Geometry: final body of the model. Coordinates: model frame, mm. Face numbers are marked on the shaded views. A direction names the side the tool comes from. Give positions to 0.01 mm unless a question says otherwise; leave off trailing zeros. Order: outer loops, then holes, each group sorted by start corner. A loop starts at its lowest first (then second) coordinate and runs counter-clockwise, first axis right, second up. Notation, with made-up numbers: (53.5, -0.5) -> (80.5, -0.5) arc R11 cw to (80.5, 3.5) -> close; hole circle Ø6 at (42.5, -27.75). An arc over 180 degrees is marked (long way). Answer in a Markdown table with one row per item. Add a question column.
Q1. Set-up query: the marked faces 1, 2, 3, 4 and 5. Return all of +Z, -Z, +X, -X, +Y, -Y with unobstructed straight access to the full face (end or side cutting, diameter ignored); none if empty.
Q2. Cut plane A-A on y = 0. Return the cut outline in (x, z).
Q3. Contact query for flat-ended pins moving along their axis: P1, Ø0.8, axis at x = 12, z = 0.5, coming from the -Y side (3 decimals); P2, Ø5, axis at x = -6, y = -8.5, coming from the +Z side; P3, Ø5, axis at x = -21.92, y = 0, coming from the +Z side; P4, Ø8, axis at x = -9, y = 2.5, coming from the -Z side. Output: stop coordinate, or through.
Q4. Cut plane B-B on x = 0. Return the cut outline in (y, z).
Q5. Cut plane C-C on y = 11. Return the cut outline in (x, z) (3 decimals).
Q6. Line query: line 1 along Y through (x, z) = (0, 0.65); line 2 along X through (y, z) = (14, 0.8) (3 decimals); line 3 along Z through (x, y) = (-16, 3). Output: solid intervals per line, ascending. Write a range as from..to.
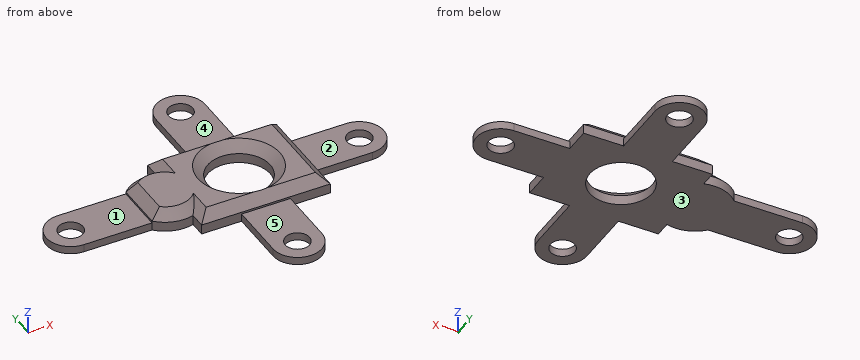
from build123d import *

# Parameters (mm, degrees)
F0_R         = 4.064
F1_DEPTH     = 2.54
F0_R_2       = 1.5875
F2_DEPTH     = 1.016
F3_T1_DEPTH  = 23.2960747894
F3_T3_DEPTH  = 19.6130747894
F3_T5_DEPTH  = 12.8820747894
F3_T10_DEPTH = 8.6144406225
F3_S11_R     = 4.6355
F3_T12_DEPTH = 6
F3_T16_ANGLE = 143.4241535748
F3_T21_ANGLE = 143.4241535748
F3_T26_DEPTH = 8.6144406225
F3_S27_R     = 4.6355
F3_T28_DEPTH = 6
F3_T35_ANGLE = 143.4241535748
F3_T39_DEPTH = 8.6144406225
F3_S40_R     = 4.6355
F3_T41_DEPTH = 6
F3_T47_DEPTH = 8.6144406225
F3_S48_R     = 4.6355
F3_T49_DEPTH = 6
F3_T52_ANGLE = 143.4241535748


# Not quite as in the source:
# - a fillet or chamfer that OpenCascade refuses, or shapes differently, is made with other operations: its cross-section is extruded or revolved along the edge and cut away or added
# - a feature names something its author has since deleted; it is built from what else it names


with BuildPart() as f1:
    # F0 (on Top) → F1 (new body)
    with BuildSketch(Plane.XY):
        Polygon((-8.382, 6.5405), (-8.382, 4.4581341669), (-8.382, -4.4581341669), (-8.382, -6.5405), (-3.175, -6.5405), (3.175, -6.5405), (8.382, -6.5405), (8.382, -3.175), (8.382, 3.175), (8.382, 6.5405), (3.175, 6.5405), (-3.175, 6.5405), align=None)
        Circle(F0_R, mode=Mode.SUBTRACT)
        with BuildLine():
            Line((-8.382, -4.4581341669), (-8.382, 4.4581341669))
            ThreePointArc((-8.382, 4.4581341669), (-10.8856754478, 4.4683224077), (-13.0294598813, 3.175))
            Line((-13.0294598813, 3.175), (-13.0294598813, -3.175))
            ThreePointArc((-13.0294598813, -3.175), (-10.8856754478, -4.4683224077), (-8.382, -4.4581341669))
        make_face()
    extrude(amount=F1_DEPTH)

    # F0 (on Top) → F2 (join)
    with BuildSketch(Plane.XY):
        with BuildLine():
            Line((-13.0294598813, -3.175), (-13.0294598813, 3.175))
            Line((-13.0294598813, 3.175), (-21.9194598813, 3.175))
            ThreePointArc((-21.9194598813, 3.175), (-25.0944598813, 0), (-21.9194598813, -3.175))
            Line((-21.9194598813, -3.175), (-13.0294598813, -3.175))
        make_face()
        with Locations((-21.9194598813, 0)):
            Circle(F0_R_2, mode=Mode.SUBTRACT)
        with BuildLine():
            Line((3.175, -6.5405), (-3.175, -6.5405))
            Line((-3.175, -6.5405), (-3.175, -14.1605))
            ThreePointArc((-3.175, -14.1605), (0, -17.3355), (3.175, -14.1605))
            Line((3.175, -14.1605), (3.175, -6.5405))
        make_face()
        with Locations((0, -14.1605)):
            Circle(F0_R_2, mode=Mode.SUBTRACT)
        with BuildLine():
            Line((-3.175, 14.1605), (-3.175, 6.5405))
            Line((-3.175, 6.5405), (3.175, 6.5405))
            Line((3.175, 6.5405), (3.175, 14.1605))
            ThreePointArc((3.175, 14.1605), (0, 17.3355), (-3.175, 14.1605))
        make_face()
        with Locations((0, 14.1605)):
            Circle(F0_R_2, mode=Mode.SUBTRACT)
        with BuildLine():
            Line((15.6725401187, 3.175), (8.382, 3.175))
            Line((8.382, 3.175), (8.382, -3.175))
            Line((8.382, -3.175), (15.6725401187, -3.175))
            ThreePointArc((15.6725401187, -3.175), (18.8475401187, 0), (15.6725401187, 3.175))
        make_face()
        with Locations((15.6725401187, 0)):
            Circle(F0_R_2, mode=Mode.SUBTRACT)
    extrude(amount=F2_DEPTH)

    # F3: chamfer of 1.27 on 9 edges, made by hand

    # F3_s2 → F3_t1 (cut)
    with BuildSketch(Plane.YZ.offset(-11.6480373947)):
        Polygon((-5.2705, 2.54), (-6.5405, 1.27), (-6.5405, 2.54), align=None)
        Polygon((6.5405, 1.27), (5.2705, 2.54), (6.5405, 2.54), align=None)
    extrude(amount=F3_T1_DEPTH, mode=Mode.SUBTRACT)

    # F3_s4 → F3_t3 (cut)
    with BuildSketch(Plane.XZ.offset(-9.8065373947)):
        Polygon((7.112, 2.54), (8.382, 1.27), (8.382, 2.54), align=None)
    extrude(amount=F3_T3_DEPTH, mode=Mode.SUBTRACT)

    # F3_s6 → F3_t5 (cut)
    with BuildSketch(Plane.XZ.offset(-6.4410373947)):
        Polygon((-11.7594598813, 2.54), (-13.0294598813, 1.27), (-13.0294598813, 2.54), align=None)
    extrude(amount=F3_T5_DEPTH, mode=Mode.SUBTRACT)


with BuildPart() as f3_tool8:
    # F3_s9 → F3_t10 (new body)
    with BuildSketch(Plane.XZ.offset(1.1920967722)):
        Polygon((-7.112, 2.54), (-8.382, 1.27), (-8.382, 2.54), align=None)
    extrude(amount=F3_T10_DEPTH)

    # F3_s11 → F3_t12 (cut, symmetric)
    with BuildSketch(Plane.XY.offset(1.9)):
        with Locations((-9.652, 0)):
            Circle(F3_S11_R)
    extrude(amount=F3_T12_DEPTH, both=True, mode=Mode.SUBTRACT)


with BuildPart() as f1_1:
    add(f1.part)

    # F3_t7: cut F3_tool8
    add(f3_tool8.part, mode=Mode.SUBTRACT)


with BuildPart() as f3_tool14:
    # F3_s15 → F3_t16 (revolve)
    with BuildSketch(Plane(origin=(-0.0239192805, 0.47989245, 0), x_dir=(0, 0, 1), z_dir=(-0.0497812044, 0.9987601472, 0))):
        Polygon((2.54, -13.005532941), (1.27, -14.275532941), (2.54, -14.275532941), align=None)
    revolve(axis=Axis((-9.652, 0, 2.54), (0, 0, 1)), revolution_arc=F3_T16_ANGLE)

    split(bisect_by=Plane.YZ.offset(-8.382), keep=Keep.BOTTOM)


with BuildPart() as f1_2:
    add(f1_1.part)

    # F3_t13: cut F3_tool14
    add(f3_tool14.part, mode=Mode.SUBTRACT)


with BuildPart() as f3_tool19:
    # F3_s20 → F3_t21 (revolve)
    with BuildSketch(Plane(origin=(-2.9748772597, 4.4568621922, 0), x_dir=(0, 0, 1), z_dir=(0.5551698459, -0.831737003, 0))):
        Polygon((1.27, 3.3924255533), (2.54, 4.6624255533), (2.54, 3.3924255533), align=None)
    revolve(axis=Axis((-9.652, 0, 2.54), (0, 0, 1)), revolution_arc=F3_T21_ANGLE)

    split(bisect_by=Plane.YZ.offset(-8.382), keep=Keep.BOTTOM)


with BuildPart() as f1_3:
    add(f1_2.part)

    # F3_t18: cut F3_tool19
    add(f3_tool19.part, mode=Mode.SUBTRACT)


with BuildPart() as f3_tool24:
    # F3_s25 → F3_t26 (new body)
    with BuildSketch(Plane.XZ.offset(-9.8065373947)):
        Polygon((-8.382, 1.27), (-7.112, 2.54), (-8.382, 2.54), align=None)
    extrude(amount=F3_T26_DEPTH)

    # F3_s27 → F3_t28 (cut, symmetric)
    with BuildSketch(Plane.XY.offset(1.9)):
        with Locations((-9.652, 0)):
            Circle(F3_S27_R)
    extrude(amount=F3_T28_DEPTH, both=True, mode=Mode.SUBTRACT)


with BuildPart() as f1_4:
    add(f1_3.part)

    # F3_t23: cut F3_tool24
    add(f3_tool24.part, mode=Mode.SUBTRACT)

    # F3_s29 → F3_t30 (revolve, cut)
    with BuildSketch(Plane.XZ):
        Polygon((5.334, 2.54), (4.064, 1.27), (4.064, 2.54), align=None)
    revolve(axis=Axis((0, 0, 2.54), (0, 0, 1)), mode=Mode.SUBTRACT)


with BuildPart() as f3_tool33:
    # F3_s34 → F3_t35 (revolve)
    with BuildSketch(Plane(origin=(-0.0239192805, 0.47989245, 0), x_dir=(0, 0, 1), z_dir=(-0.0497812044, 0.9987601472, 0))):
        Polygon((2.54, -13.005532941), (1.27, -14.275532941), (2.54, -14.275532941), align=None)
    revolve(axis=Axis((-9.652, 0, 2.54), (0, 0, 1)), revolution_arc=F3_T35_ANGLE)

    split(bisect_by=Plane.YZ.offset(-8.382), keep=Keep.TOP)


with BuildPart() as f3_tool37:
    # F3_s38 → F3_t39 (new body)
    with BuildSketch(Plane.XZ.offset(1.1920967722)):
        Polygon((-7.112, 2.54), (-8.382, 1.27), (-8.382, 2.54), align=None)
    extrude(amount=F3_T39_DEPTH)

    # F3_s40 → F3_t41 (intersect, symmetric)
    with BuildSketch(Plane.XY.offset(1.9)):
        with Locations((-9.652, 0)):
            Circle(F3_S40_R)
    extrude(amount=F3_T41_DEPTH, both=True, mode=Mode.INTERSECT)


with BuildPart() as f3_tool33_1:
    add(f3_tool33.part)

    # F3_t42: intersect F3_tool37
    add(f3_tool37.part, mode=Mode.INTERSECT)


with BuildPart() as f1_5:
    add(f1_4.part)

    # F3_t31: cut F3_tool33
    add(f3_tool33_1.part, mode=Mode.SUBTRACT)


with BuildPart() as f3_tool45:
    # F3_s46 → F3_t47 (new body)
    with BuildSketch(Plane.XZ.offset(-9.8065373947)):
        Polygon((-8.382, 1.27), (-7.112, 2.54), (-8.382, 2.54), align=None)
    extrude(amount=F3_T47_DEPTH)

    # F3_s48 → F3_t49 (intersect, symmetric)
    with BuildSketch(Plane.XY.offset(1.9)):
        with Locations((-9.652, 0)):
            Circle(F3_S48_R)
    extrude(amount=F3_T49_DEPTH, both=True, mode=Mode.INTERSECT)


with BuildPart() as f3_tool50:
    # F3_s51 → F3_t52 (revolve)
    with BuildSketch(Plane(origin=(-2.9748772597, 4.4568621922, 0), x_dir=(0, 0, 1), z_dir=(0.5551698459, -0.831737003, 0))):
        Polygon((1.27, 3.3924255533), (2.54, 4.6624255533), (2.54, 3.3924255533), align=None)
    revolve(axis=Axis((-9.652, 0, 2.54), (0, 0, 1)), revolution_arc=F3_T52_ANGLE)

    split(bisect_by=Plane.YZ.offset(-8.382), keep=Keep.TOP)


with BuildPart() as f3_tool45_1:
    add(f3_tool45.part)

    # F3_t54: intersect F3_tool50
    add(f3_tool50.part, mode=Mode.INTERSECT)


with BuildPart() as f1_6:
    add(f1_5.part)

    # F3_t43: cut F3_tool45
    add(f3_tool45_1.part, mode=Mode.SUBTRACT)


solid = f1_6.part
Completed:
| question | item | result |
|---|---|---|
| 1 | face 1 | +Z, -X, +Y, -Y |
| 1 | face 2 | +Z, +X, +Y, -Y |
| 1 | face 3 | -Z, +X, -X, +Y, -Y |
| 1 | face 4 | +Z, +X, -X, +Y |
| 1 | face 5 | +Z, +X, -X, -Y |
| 2 | outline | (-25.09, 0) -> (-23.51, 0) -> (-23.51, 1.02) -> (-25.09, 1.02) -> close; (-20.33, 0) -> (-4.06, 0) -> (-4.06, 1.27) -> (-5.33, 2.54) -> (-11.76, 2.54) -> (-13.03, 1.27) -> (-13.03, 1.02) -> (-20.33, 1.02) -> close; (4.06, 0) -> (14.09, 0) -> (14.09, 1.02) -> (8.38, 1.02) -> (8.38, 1.27) -> (7.11, 2.54) -> (5.33, 2.54) -> (4.06, 1.27) -> close; (17.26, 0) -> (18.85, 0) -> (18.85, 1.02) -> (17.26, 1.02) -> close |
| 3 | P1 | stops at y = -3.175 |
| 3 | P2 | stops at z = 1.81 |
| 3 | P3 | stops at z = 1.02 |
| 3 | P4 | stops at z = 0 |
| 4 | outline | (-17.34, 0) -> (-15.75, 0) -> (-15.75, 1.02) -> (-17.34, 1.02) -> close; (-12.57, 0) -> (-4.06, 0) -> (-4.06, 1.27) -> (-5.3, 2.51) -> (-6.54, 1.27) -> (-6.54, 1.02) -> (-12.57, 1.02) -> close; (4.06, 0) -> (12.57, 0) -> (12.57, 1.02) -> (6.54, 1.02) -> (6.54, 1.27) -> (5.3, 2.51) -> (4.06, 1.27) -> close; (15.75, 0) -> (17.34, 0) -> (17.34, 1.02) -> (15.75, 1.02) -> close |
| 5 | outline | (-3.175, 0) -> (3.175, 0) -> (3.175, 1.016) -> (-3.175, 1.016) -> close |
| 6 | line 1 | y = -17.34..-15.75, -12.57..-4.06, 4.06..12.57, 15.75..17.34 |
| 6 | line 2 | x = -3.175..-1.579, 1.579..3.175 |
| 6 | line 3 | z = 0..1.02 |
